from build123d import *

# Parameters (mm, degrees)
F1_DEPTH = 100
F2_W     = 20
F2_H     = 30
F3_DEPTH = 1
F4_R     = 4.99999
F5_R     = 2


# Not quite as in the source:
# - a fillet or chamfer is up to 0.001 mm smaller than in the source, because OpenCascade refuses the exact size


with BuildPart() as f1:
    # F0 (on Right) → F1 (new body)
    with BuildSketch(Plane.YZ):
        Polygon((-4, 7), (-5, 7), (-5, 0), (5, 0), (5, 7), (4, 7), (4, 1), (-4, 1), align=None)
    extrude(amount=F1_DEPTH)

    # F2 (on Top) → F3 (join)
    with BuildSketch(Plane.XY):
        with Locations((20, 0)):
            Rectangle(F2_W, F2_H)
        with Locations((80, 0)):
            Rectangle(F2_W, F2_H)
    extrude(amount=F3_DEPTH)

    # F4 (radius 5 in the source; OpenCascade refuses exactly that, so slightly less here)
    f4_edges = [f1.edges().sort_by_distance(p)[0] for p in [
        (20, -5, 1),
        (80, -5, 1),
        (20, 5, 1),
        (80, 5, 1),
        (10, -15, 0.5),
        (30, -15, 0.5),
        (70, -15, 0.5),
        (90, -15, 0.5),
        (10, 15, 0.5),
        (30, 15, 0.5),
        (70, 15, 0.5),
        (90, 15, 0.5),
    ]]
    fillet(f4_edges, radius=F4_R)

    # F5
    f5_edges = [f1.edges().sort_by_distance(p)[0] for p in [
        (50, 4, 1),
        (50, -4, 1),
    ]]
    fillet(f5_edges, radius=F5_R)


solid = f1.part
For this review, take the finished solid that the model builds, in its own axes (mm). A direction names the side the tool comes from. Give positions to 0.01 mm unless a question says otherwise; leave off trailing zeros. Order: outer loops, then holes, each group sorted by start corner. A loop starts at its lowest first (then second) coordinate and runs counter-clockwise, first axis right, second up. Notation, with made-up numbers: (76.25, -22) - (104.25, -22) arc R35 ccw to (104.25, 17) - close; hole circle Ø10 at (77, 45). An arc over 180 degrees is marked (long way). Answer as a JSON object with one key per item and string values. Group by question number.
Item 1: Machinability: for faces 4 (the cylindrical face through (71.5, -13.57, 0.51)), 5 (the cylindrical face through (28.5, 13.57, 0.51)), 6 (the flat face through (20, -12, 1)), 7 (the flat face through (49, 4, 5)), which of the approach directions +Z, -Z, +X, -X, +Y, -Y give a long, thin tool a straight path to every point of the face, cutting with its end or side? Answer none if there is none.
Item 2: Take a section at A-A on y = -9. Give the boundary of the cut face in (x, z), and give its area (3 significant figures).
Item 3: Wall thickness on line 1 along Y through (x, z) = (49, 3); line 2 along Z through (x, y) = (77, 11.25); line 3 along Z through (x, y) = (78, 7): over which ranges is each line inside the solid? List them lowest first.
Item 4: Take a section at C-C on z = 5. Give the boundary of the cut face in (x, y), and give its area (3 significant figures).
Item 5: Take a section at B-B on x = 47. Give the boundary of the cut face in (y, z), and give its area (3 significant figures).
Item 6: Clearance check with flat-ended pins moving along their axes: pin 1 Ø1.5 at (x, y) = (20, 12.5) entering from +Z; pin 2 Ø1.2 at (x, z) = (58, 5.5) entering from +Y; pin 3 Ø2.5 at (y, z) = (-7.5, 2) entering from +X; pin 4 Ø5 at (x, y) = (50, -9.5) entering from -Z. State where each tip first meets the part, or that it passes through.
Item 7: Take a section at D-D on y = 11.75. Give the boundary of the cut face in (x, z).
Item 8: Draft analysis for pull direction X (two halves, no side actions). For faces 1 (the flat face through (90, 6.9, 1.6)), 2 (the cylindrical face through (71.43, 13.5, 0.51)), 3 (the cylindrical face through (50.7, 3.4, 1.57)), state which applies: pulls with the +X half, pulls with the -X half, needs draft (parallel to the pull), parting line crosses it, or undercut.
Reported:
{
 "1": {"face 4": "+Z, -Z, -Y", "face 5": "+Z, -Z, +Y", "face 6": "+Z, +X, -X, -Y", "face 7": "+Z, +X, -X"},
 "2": {"outline": "(10, 0) - (30, 0) - (30, 1.1) - (10, 1.1) - close; (70, 0) - (90, 0) - (90, 1.1) - (70, 1.1) - close", "area": "44.0 mm^2"},
 "3": {"line 1": "-5 to -4, 4 to 5", "line 2": "0 to 1", "line 3": "0 to 2"},
 "4": {"outline": "(0, -5) - (10, -5) - (10, -5.1) - (30, -5.1) - (30, -5) - (70, -5) - (70, -5.1) - (90, -5.1) - (90, -5) - (100, -5) - (100, -4) - (0, -4) - close; (0, 4) - (100, 4) - (100, 5) - (90, 5) - (90, 5.1) - (70, 5.1) - (70, 5) - (30, 5) - (30, 5.1) - (10, 5.1) - (10, 5) - (0, 5) - close", "area": "208 mm^2"},
 "5": {"outline": "(-5, 0) - (5, 0) - (5, 7) - (4, 7) - (4, 3) arc R2 cw to (2, 1) - (-2, 1) arc R2 cw to (-4, 3) - (-4, 7) - (-5, 7) - close", "area": "23.7 mm^2"},
 "6": {"pin 1": "z = 1", "pin 2": "y = 5", "pin 3": "x = 90", "pin 4": "through"},
 "7": {"outline": "(10.32, 0) - (29.68, 0) - (29.68, 1) - (10.32, 1) - close; (70.32, 0) - (89.68, 0) - (89.68, 1) - (70.32, 1) - close"},
 "8": {"face 1": "pulls with the +X half", "face 2": "undercut", "face 3": "needs draft"}
}
